Geometry: final body of the model. Coordinates: model frame, mm. A direction names the side the tool comes from. Give positions to 0.01 mm unless a question says otherwise; leave off trailing zeros. Order: outer loops, then holes, each group sorted by start corner. A loop starts at its lowest first (then second) coordinate and runs counter-clockwise, first axis right, second up. Notation, with made-up numbers: (76.5, 32) -> (125.5, 32) arc R20 cw to (125.5, 56) -> close; hole circle Ø9 at (30.5, 36). An arc over 180 degrees is marked (long way). Answer in a Markdown table with one row per item. Add a question column.
Q1. Cut plane B-B on x = 0. Return the cut outline in (y, z).
Q2. Set-up query: faces 1 (the face through (2.753, 31.306, -62.924)), 2 (the face through (34, -19, 21.4)), 3 (the face through (-1, -38.1, -16)). Return all of +Z, -Z, +X, -X, +Y, -Y with unobstructed straight access to the full face (end or side cutting, diameter ignored); none if empty.
Q3. Line query: line 1 along X through (y, z) = (-9, -2.5); line 2 along X through (y, z) = (-11, -33.5); line 3 along Y through (x, z) = (-56.5, -34). Output: solid intervals per line, ascending. Write a range as from..to.
Q4. Pull-direction query (X, two-part tool) for faces 4 (the face through (0, 63.5, -50)), 5 (the face through (-60.47, -18.783, -46.367)), 6 (the face through (-38.73, -19.32, -42.75)), 7 (the face through (-40.99, 31.31, 0.56)); classes: +X half, -X half, draft (parallel to the pull), parting line (faces both ways), or undercut.
Q5. Cut plane A-A on z = 0. Return the cut outline in (x, y).
Q6. Cut plane C-C on z = -29. Return the cut outline in (x, y).
Q7. Contact query for flat-ended pins moving along their axis: P1, Ø3, axis at y = -12, z = -52.5, coming from the -X side; P2, Ø10, axis at y = -15, z = -34.5, coming from the +X side; P3, Ø8, axis at y = -24, z = 24, coming from the -X side; P4, Ø1.5, axis at x = 46.5, z = -12, coming from the +Y side. Output: stop coordinate, or through.
Q8. Cut plane D-D on y = -14. Return the cut outline in (x, z).
from build123d import *

# Parameters (mm, degrees)
F0_R      = 76.2
F1_DEPTH  = 38.1
F3_R      = 15.24
F4_DEPTH  = 38.1
F5_DEPTH  = 50.8
F7_DEPTH  = 38.1
F8_R      = 12.7
F9_DEPTH  = 63.5
F10_W     = 33.02
F10_H     = 20.32
F11_DEPTH = 50.8
F13_DEPTH = 38.1
F14_DEPTH = 38.1
F15_DEPTH = 38.1


with BuildPart() as f1:
    # F0 (on Front) → F1 (new body)
    with BuildSketch(Plane.XZ):
        Circle(F0_R)
    extrude(amount=F1_DEPTH)

    # F3 (on face) → F4 (cut)
    with BuildSketch(Plane.XZ.offset(38.1)):
        with Locations((-33.264, 40.697999)):
            Circle(F3_R)
    extrude(amount=-F4_DEPTH, mode=Mode.SUBTRACT)

    # F2 (on face) → F5 (cut)
    with BuildSketch(Plane.XZ.offset(38.1)):
        Polygon((34.082881, 51.879571), (18.842881, 21.399571), (49.322881, 21.399571), align=None)
    extrude(amount=-F5_DEPTH, mode=Mode.SUBTRACT)

    # F6 (on face) → F7 (cut)
    with BuildSketch(Plane.XZ.offset(38.1)):
        Polygon((15.24, 15.24), (0, 15.24), (-15.24, 15.24), (-15.24, -15.24), (0, -15.24), (15.24, -15.24), align=None)
    extrude(amount=-F7_DEPTH, mode=Mode.SUBTRACT)

    # F8 (on face) → F9 (join)
    with BuildSketch(Plane(origin=(0, 0, 0), x_dir=(-1, 0, 0), z_dir=(0, 1, 0))):
        with Locations((0, 53.110374)):
            Circle(F8_R)
        with Locations((0, -50.526001)):
            Circle(F8_R)
        with Locations((53.675998, 0)):
            Circle(F8_R)
        with Locations((-52.416001, 0)):
            Circle(F8_R)
    extrude(amount=F9_DEPTH)

    # F10 (on face) → F11 (cut)
    with BuildSketch(Plane.XZ.offset(38.1)):
        with Locations((35.620325, -34.899539)):
            Rectangle(F10_W, F10_H)
    extrude(amount=-F11_DEPTH, mode=Mode.SUBTRACT)

    # F12 (on face) → F13 (cut)
    with BuildSketch(Plane.XZ.offset(38.1)):
        Polygon((-20.681122, -34.290014), (-34.688334, -23.338923), (-45.639425, -37.346136), (-31.632213, -48.297227), align=None)
    extrude(amount=F13_DEPTH, mode=Mode.SUBTRACT)

    # F12 (on face) → F14 (cut)
    with BuildSketch(Plane.XZ.offset(38.1)):
        Polygon((-20.681122, -34.290014), (-34.688334, -23.338923), (-45.639425, -37.346136), (-31.632213, -48.297227), align=None)
    extrude(amount=-F14_DEPTH, mode=Mode.SUBTRACT)

    # F12 (on face) → F15 (cut)
    with BuildSketch(Plane.XZ.offset(38.1)):
        Polygon((-20.681122, -34.290014), (-34.688334, -23.338923), (-45.639425, -37.346136), (-31.632213, -48.297227), align=None)
    extrude(amount=-F15_DEPTH, mode=Mode.SUBTRACT)


solid = f1.part
Completed:
| question | item | result |
|---|---|---|
| 1 | outline | (-38.1, -76.2) -> (0, -76.2) -> (0, -63.23) -> (63.5, -63.23) -> (63.5, -37.83) -> (0, -37.83) -> (0, -15.24) -> (-38.1, -15.24) -> close; (-38.1, 15.24) -> (0, 15.24) -> (0, 40.41) -> (63.5, 40.41) -> (63.5, 65.81) -> (0, 65.81) -> (0, 76.2) -> (-38.1, 76.2) -> close |
| 2 | face 1 | +Y |
| 2 | face 2 | +Y, -Y |
| 2 | face 3 | +Z, -Z, +X, -X, -Y |
| 3 | line 1 | x = -76.16..-15.24, 15.24..76.16 |
| 3 | line 2 | x = -68.44..-42.63, -21.69..19.11, 52.13..68.44 |
| 3 | line 3 | y = -38.1..0 |
| 4 | face 4 | draft |
| 4 | face 5 | parting line |
| 4 | face 6 | undercut |
| 4 | face 7 | undercut |
| 5 | outline | (-76.2, -38.1) -> (-15.24, -38.1) -> (-15.24, 0) -> (-40.98, 0) -> (-40.98, 63.5) -> (-66.38, 63.5) -> (-66.38, 0) -> (-76.2, 0) -> close; (15.24, -38.1) -> (76.2, -38.1) -> (76.2, 0) -> (65.12, 0) -> (65.12, 63.5) -> (39.72, 63.5) -> (39.72, 0) -> (15.24, 0) -> close |
| 6 | outline | (-70.47, -38.1) -> (-39.11, -38.1) -> (-39.11, 0) -> (-70.47, 0) -> close; (-27.45, -38.1) -> (19.11, -38.1) -> (19.11, 0) -> (-27.45, 0) -> close; (52.13, -38.1) -> (70.47, -38.1) -> (70.47, 0) -> (52.13, 0) -> close |
| 7 | P1 | stops at x = -56.62 |
| 7 | P2 | stops at x = 70.26 |
| 7 | P3 | stops at x = -73.53 |
| 7 | P4 | stops at y = 63.5 |
| 8 | outline | circle Ø152.4 at (0, 0); hole circle Ø30.48 at (-33.26, 40.7); hole (-45.64, -37.35) -> (-31.63, -48.3) -> (-20.68, -34.29) -> (-34.69, -23.34) -> close; hole (-15.24, -15.24) -> (15.24, -15.24) -> (15.24, 15.24) -> (-15.24, 15.24) -> close; hole (18.84, 21.4) -> (49.32, 21.4) -> (34.08, 51.88) -> close; hole (19.11, -45.06) -> (52.13, -45.06) -> (52.13, -24.74) -> (19.11, -24.74) -> close |
